Could you check a few things on this model? Use its own coordinates, in mm. Coordinates: 2 decimals unless noted, no trailing zeros. Order: outer loops, then holes, each group sorted by start corner. A loop starts at its lowest first (then second) coordinate and runs counter-clockwise, first axis right, second up. Notation, with made-up numbers: (-39.5, -4.5) -> (11.5, -4.5) arc R13 cw to (11.5, 17.5) -> close; hole circle Ø4 at (15.25, -26.75). An arc over 180 degrees is marked (long way). Use a Markdown table: item, result. Add a question column.
1) If we section it at B-B (x = 217.25): Write out the boundary of the cut face in (y, z).
2) Will these pins go through, and if not, where does the flat tip stop? pin 1 Ø1.2 at (x, z) = (3, 2) entering from +Y; pin 2 Ø1.2 at (x, z) = (22.5, 1.5) entering from -Y.
3) If we section it at D-D (z = 0.9): Give the number of separate pieces and of enclosed holes in the cut face, plus the area to 3 significant figures.
4) If we section it at A-A (y = 61.35): Write out the boundary of the cut face in (x, z).
5) If we section it at C-C (y = 159.5): Write out the boundary of the cut face in (x, z), plus the area to 3 significant figures.
6) If I drill on L1, parallel to Y at x = 313.25, z = 2.7; L2, parallel to Y at x = 483.5, z = 2.1; L3, parallel to X at y = 163.5, z = 3.65, over which ranges is the centre line in solid material (lowest first)? Write a range as [from, to].
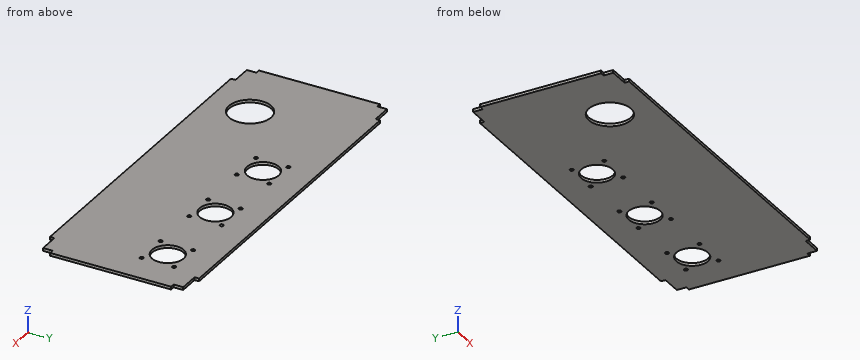
Autodesk Inventor part; units mm, degrees
ref_plane "YZ Plane" through (0, 0, 0) normal (1, 0, 0) x (0, 1, 0)
ref_plane "XZ Plane" through (0, 0, 0) normal (0, 1, 0) x (-1, 0, 0)
ref_plane "XY Plane" through (0, 0, 0) normal (0, 0, 1) x (1, 0, 0)
sketch "Skizze1" plane through (0, 0, 0) normal (0, 0, 1) x (1, 0, 0)
  line L0 (0, 0) -> (526.5, 0)
  line L1 (526.5, 0) -> (526.5, 212.5)
  line L2 (526.5, 212.5) -> (0, 212.5)
  line L3 (0, 212.5) -> (0, 0)
  line L4 (0, 212.5) -> (35, 212.5)
  line L5 (35, 212.5) -> (35, 206.15)
  line L6 (35, 206.15) -> (0, 206.15)
  line L7 (0, 206.15) -> (0, 212.5)
  line L8 (0, 212.5) -> (6.35, 212.5)
  line L9 (6.35, 212.5) -> (6.35, 192.5)
  line L10 (6.35, 192.5) -> (0, 192.5)
  line L11 (0, 192.5) -> (0, 212.5)
  line L12 (0, 106.25) -> (526.5, 106.25) construction
  line L13 (263.25, 212.5) -> (263.25, 0) construction
  line L14 (0, 0) -> (35, 0)
  line L15 (35, 0) -> (35, 6.35)
  line L16 (35, 6.35) -> (0, 6.35)
  line L17 (0, 6.35) -> (0, 0)
  line L18 (0, 0) -> (6.35, 0)
  line L19 (6.35, 0) -> (6.35, 20)
  line L20 (6.35, 20) -> (0, 20)
  line L21 (0, 20) -> (0, 0)
  line L22 (526.5, 212.5) -> (526.5, 0)
  line L23 (526.5, 212.5) -> (491.5, 212.5)
  line L24 (491.5, 212.5) -> (491.5, 206.15)
  line L25 (491.5, 206.15) -> (526.5, 206.15)
  line L26 (526.5, 206.15) -> (526.5, 212.5)
  line L27 (526.5, 212.5) -> (520.15, 212.5)
  line L28 (520.15, 212.5) -> (520.15, 192.5)
  line L29 (520.15, 192.5) -> (526.5, 192.5)
  line L30 (526.5, 192.5) -> (526.5, 212.5)
  line L31 (526.5, 0) -> (520.15, 0)
  line L32 (526.5, 0) -> (491.5, 0)
  line L33 (491.5, 0) -> (491.5, 6.35)
  line L34 (491.5, 6.35) -> (526.5, 6.35)
  line L35 (520.15, 0) -> (520.15, 20)
  line L36 (526.5, 6.35) -> (526.5, 0)
  line L37 (520.15, 20) -> (526.5, 20)
  line L38 (526.5, 20) -> (526.5, 0)
  point P0 (526.5, 192.5)
  point P1 (520.15, 206.15)
  point P2 (491.5, 212.5)
  point P3 (6.35, 206.15)
  point P4 (0, 192.5)
  point P5 (0, 20)
  point P6 (6.35, 6.35)
  point P7 (491.5, 0)
  point P8 (520.15, 6.35)
  point P9 (526.5, 20)
  dimension "d0" = 526.5
  dimension "d1" = 212.5
  dimension "d2" = 35
  dimension "d3" = 6.35
  dimension "d4" = 6.35
  dimension "d5" = 20
extrude "Extrusion1" add sketch "Skizze1" along normal blind 4 contours L15 L16 L19 L20 L3 L10 L9 L6 L5 L2 L24 L25 L28 L29 L1 L37 L35 L34 L33 L0
sketch "Skizze3" plane through (0, 0, 4) normal (0, 0, 1) x (1, 0, 0)
  circle A0 centre (217.25, 148.65) radius 22.5
  circle A1 centre (337.25, 148.65) radius 22.5
  circle A2 centre (457.25, 148.65) radius 22.5
  circle A3 centre (95.35, 61.35) radius 30
  line L0 (520.15, 206.15) -> (491.5, 206.15)
  line L1 (520.15, 192.5) -> (520.15, 206.15)
  line L2 (6.35, 20) -> (6.35, 6.35)
  line L3 (6.35, 6.35) -> (35, 6.35)
  point P0 (0, 0)
  dimension "d19" = 45
  dimension "d20" = 45
  dimension "d21" = 45
  dimension "d22" = 60
  dimension "d23" = 120
  dimension "d24" = 120
  dimension "d25" = 57.5
  dimension "d26" = 62.9
  dimension "d27" = 89
  dimension "d28" = 55
extrude "Extrusion3" cut sketch "Skizze3" against normal blind 10
sketch "Skizze4" plane through (0, 0, 4) normal (0, 0, 1) x (1, 0, 0)
  circle A0 centre (193.25, 171.1) radius 2.6
  circle A1 centre (241.25, 171.1) radius 2.6
  circle A2 centre (241.25, 124.85) radius 2.6
  circle A3 centre (193.25, 124.85) radius 2.6
  circle A4 centre (217.25, 148.65) radius 22.5
  line L0 (491.5, 212.5) -> (35, 212.5)
  line L1 (277.25, 212.5) -> (277.25, 70.6491) construction
  line L2 (397.25, 212.5) -> (397.25, 70.6491) construction
  circle A5 centre (337.25, 148.65) radius 22.5
  circle A6 centre (361.25, 171.1) radius 2.6
  circle A7 centre (313.25, 171.1) radius 2.6
  circle A8 centre (313.25, 124.85) radius 2.6
  circle A9 centre (361.25, 124.85) radius 2.6
  circle A10 centre (481.25, 171.1) radius 2.6
  circle A11 centre (481.25, 124.85) radius 2.6
  circle A12 centre (433.25, 171.1) radius 2.6
  circle A13 centre (433.25, 124.85) radius 2.6
  point P0 (0, 0)
  point P1 (337.25, 148.65)
  point P2 (457.25, 148.65)
  point P3 (457.25, 148.65)
  dimension "d31" = 5.2
  dimension "d32" = 5.2
  dimension "d33" = 5.2
  dimension "d34" = 5.2
  dimension "d35" = 48
  dimension "d36" = 46.25
  dimension "d37" = 24
  dimension "d38" = 24
  dimension "d39" = 22.45
  dimension "d40" = 23.8
  dimension "d43" = 60
  dimension "d44" = 60
extrude "Extrusion4" cut sketch "Skizze4" against normal blind 10 contours A0 | A1 | A2 | A3 | A6 | A7 | A8 | A9 | A10 | A11 | A12 | A13
properties part number "103.015.01_Abdeckung_Gestell_oben" material "PMMA-Kunststoff"
Answer sheet:
| question | item | result |
|---|---|---|
| 1 | outline | (0, 0) -> (126.15, 0) -> (126.15, 4) -> (0, 4) -> close; (171.15, 0) -> (212.5, 0) -> (212.5, 4) -> (171.15, 4) -> close |
| 2 | pin 1 | y = 192.5 |
| 2 | pin 2 | y = 6.35 |
| 3 | separate pieces | 1 |
| 3 | enclosed holes | 16 |
| 3 | area | 103,000 mm2 |
| 4 | outline | (0, 0) -> (65.35, 0) -> (65.35, 4) -> (0, 4) -> close; (125.35, 0) -> (526.5, 0) -> (526.5, 4) -> (125.35, 4) -> close |
| 5 | outline | (0, 0) -> (197.54, 0) -> (197.54, 4) -> (0, 4) -> close; (236.96, 0) -> (317.54, 0) -> (317.54, 4) -> (236.96, 4) -> close; (356.96, 0) -> (437.54, 0) -> (437.54, 4) -> (356.96, 4) -> close; (476.96, 0) -> (526.5, 0) -> (526.5, 4) -> (476.96, 4) -> close |
| 5 | area | 1,630 mm2 |
| 6 | L1 | [0, 122.25], [127.45, 168.5], [173.7, 212.5] |
| 6 | L2 | [0, 123.55], [126.15, 169.8], [172.4, 212.5] |
| 6 | L3 | [0, 200.35], [234.15, 320.35], [354.15, 440.35], [474.15, 526.5] |
